```python
from build123d import *
from build123d.topology import SkipClean

# Parameters (mm, degrees)
SKETCH1_R           = 37.25
BOSS_EXTRUDE1_DEPTH = 1.2
SKETCH2_R           = 20.1
SKETCH2_W           = 26.3
SKETCH2_H           = 19.35
SKETCH2_W_2         = 15.8
SKETCH2_H_2         = 1.8
BOSS_EXTRUDE3_DEPTH = 2
SKETCH2_5_R         = 22.5
SKETCH2_5_R_2       = 20.1
BOSS_EXTRUDE4_DEPTH = 5.6
SKETCH2_7_R         = 22.5
SKETCH2_7_R_2       = 20.1
SKETCH2_7_W         = 26.3
SKETCH2_7_H         = 19.35
SKETCH2_7_W_2       = 15.8
SKETCH2_7_H_2       = 1.8
CUT_EXTRUDE1_DEPTH  = 55.800866781
CUT_EXTRUDE2_DEPTH  = 54.52919764
SKETCH8_R           = 1.5
CUT_EXTRUDE3_DEPTH  = 55.283837374
CUT_EXTRUDE4_DEPTH  = 54.52919764
CUT_EXTRUDE5_REACH  = 74.76


with BuildPart() as part:
    # Sketch1 → Boss-Extrude1 (new body)
    with BuildSketch(Plane(origin=(0, 0, 0), x_dir=(1, 0, 0), z_dir=(0, 1, 0))):
        with Locations(Location((0, 0, 0), (0, 0, 270))):
            Circle(SKETCH1_R)
    extrude(amount=BOSS_EXTRUDE1_DEPTH)

    # Sketch2 → Boss-Extrude3 (add)
    # profile 1 of 3: a face of its own
    with BuildSketch(Plane(origin=(0, 1.2, 0), x_dir=(1, 0, 0), z_dir=(0, 1, 0))):
        with Locations(Location((0, 0, 0), (0, 0, 270))):
            Circle(SKETCH2_R)
        with Locations((-2.45, 1.2)):
            Rectangle(SKETCH2_W, SKETCH2_H, mode=Mode.SUBTRACT)
    # profile 2 of 3: a face of its own
    with BuildSketch(Plane(origin=(0, 1.2, 0), x_dir=(1, 0, 0), z_dir=(0, 1, 0))):
        with Locations((0, 7.175)):
            Rectangle(SKETCH2_W_2, SKETCH2_H_2)
    # profile 3 of 3: a face of its own
    with BuildSketch(Plane(origin=(0, 1.2, 0), x_dir=(1, 0, 0), z_dir=(0, 1, 0))):
        with Locations((0, -7.175)):
            Rectangle(SKETCH2_W_2, SKETCH2_H_2)
    extrude(amount=BOSS_EXTRUDE3_DEPTH)

    # Sketch2<5> → Boss-Extrude4 (add)
    with BuildSketch(Plane(origin=(0, 1.2, 0), x_dir=(1, 0, 0), z_dir=(0, 1, 0))):
        with Locations(Location((0, 0, 0), (0, 0, 270))):
            Circle(SKETCH2_5_R)
        with Locations(Location((0, 0, 0), (0, 0, 270))):
            Circle(SKETCH2_5_R_2, mode=Mode.SUBTRACT)
    extrude(amount=BOSS_EXTRUDE4_DEPTH)


with BuildPart() as body_2:
    # Loft1: read off the stored shape, not the designer's step
    # Loft1 outline → Loft1 (revolve)
    with BuildSketch(Plane.XY):
        Polygon((0, 16.3), (0, 1.2), (37.25, 1.2), (24.5, 16.3), align=None)
    revolve(axis=Axis((0, 0, 0), (0, 1, 0)))

    # Sketch2<7> → Cut-Extrude1 (cut, through all)
    # profile 1 of 5: a face of its own
    with BuildSketch(Plane(origin=(0, 1.2, 0), x_dir=(1, 0, 0), z_dir=(0, 1, 0))):
        with Locations(Location((0, 0, 0), (0, 0, 90))):
            Circle(SKETCH2_7_R)
        with Locations(Location((0, 0, 0), (0, 0, 270))):
            Circle(SKETCH2_7_R_2, mode=Mode.SUBTRACT)
    # profile 2 of 5: a face of its own
    with BuildSketch(Plane(origin=(0, 1.2, 0), x_dir=(1, 0, 0), z_dir=(0, 1, 0))):
        with Locations(Location((0, 0, 0), (0, 0, 270))):
            Circle(SKETCH2_7_R_2)
        with Locations((-2.45, 1.2)):
            Rectangle(SKETCH2_7_W, SKETCH2_7_H, mode=Mode.SUBTRACT)
    # profile 3 of 5: a face of its own
    with BuildSketch(Plane(origin=(0, 1.2, 0), x_dir=(1, 0, 0), z_dir=(0, 1, 0))):
        with Locations((-2.45, 1.2)):
            Rectangle(SKETCH2_7_W, SKETCH2_7_H)
        with Locations((0, 7.175)):
            Rectangle(SKETCH2_7_W_2, SKETCH2_7_H_2, mode=Mode.SUBTRACT)
        with Locations((0, -7.175)):
            Rectangle(SKETCH2_7_W_2, SKETCH2_7_H_2, mode=Mode.SUBTRACT)
    # profile 4 of 5: a face of its own
    with BuildSketch(Plane(origin=(0, 1.2, 0), x_dir=(1, 0, 0), z_dir=(0, 1, 0))):
        with Locations((0, 7.175)):
            Rectangle(SKETCH2_7_W_2, SKETCH2_7_H_2)
    # profile 5 of 5: a face of its own
    with BuildSketch(Plane(origin=(0, 1.2, 0), x_dir=(1, 0, 0), z_dir=(0, 1, 0))):
        with Locations((0, -7.175)):
            Rectangle(SKETCH2_7_W_2, SKETCH2_7_H_2)
    extrude(amount=CUT_EXTRUDE1_DEPTH, mode=Mode.SUBTRACT)


with BuildPart() as part_1:
    add(part.part)

    # Combine1: union body 2
    add(body_2.part)

    # Sketch7 → Cut-Extrude2 (cut, through all)
    with BuildSketch(Plane(origin=(0, 6.8, 0), x_dir=(1, 0, 0), z_dir=(0, 1, 0))):
        with BuildLine():
            Line((-7.9, 10.875), (-7.9, -8.475))
            Line((-7.9, -8.475), (-20.842849493, -8.475))
            ThreePointArc((-20.842849493, -8.475), (-22.460675412, 1.329684188), (-19.69731898, 10.875))
            Line((-19.69731898, 10.875), (-7.9, 10.875))
        make_face()
    extrude(amount=-CUT_EXTRUDE2_DEPTH, mode=Mode.SUBTRACT)

    # Sketch8 → Cut-Extrude3 (cut, through all)
    with BuildSketch(Plane(origin=(0, 3.2, 0), x_dir=(1, 0, 0), z_dir=(0, 1, 0))):
        with Locations(Location((0, 14, 0), (0, 0, 270))):
            Circle(SKETCH8_R)
        with Locations(Location((0, -14, 0), (0, 0, 270))):
            Circle(SKETCH8_R)
    extrude(amount=-CUT_EXTRUDE3_DEPTH, mode=Mode.SUBTRACT)

    # Sketch9 → Cut-Extrude4 (cut, through all)
    with SkipClean():  # the faces are left unmerged after this step: merging them gives an invalid solid
        with BuildSketch(Plane(origin=(0, 6.8, 0), x_dir=(1, 0, 0), z_dir=(0, 1, 0))):
            with BuildLine():
                Line((7.9, 10.875), (7.9, -8.475))
                Line((7.9, -8.475), (20.842849493, -8.475))
                ThreePointArc((20.842849493, -8.475), (22.460675412, 1.329684188), (19.69731898, 10.875))
                Line((19.69731898, 10.875), (7.9, 10.875))
            make_face()
        extrude(amount=-CUT_EXTRUDE4_DEPTH, mode=Mode.SUBTRACT)

    # Chamfer1: read off the stored shape, not the designer's step
    # Chamfer1 outline → Chamfer1 (revolve, cut)
    with SkipClean():  # the faces are left unmerged after this step: merging them gives an invalid solid
        with BuildSketch(Plane.XY):
            Polygon((37.25, 1.806111173), (36.738217387, 1.806111173), (37.25, 0.4), align=None)
        revolve(axis=Axis((0, 0, 0), (0, 1, 0)), mode=Mode.SUBTRACT)

    # Cut-Extrude5: up to this cone (the profile starts outside it)
    with SkipClean():  # the faces are left unmerged after this step: merging them gives an invalid solid
        cut_extrude5_end = Plane(origin=(0, 13.007369, 0), z_dir=(0, -1, 0)).offset(-31.6883035) * Cone(1e-06, 112.896593677, 133.704984453, align=(Align.CENTER, Align.CENTER, Align.MIN), mode=Mode.PRIVATE)
        # Sketch10 → Cut-Extrude5 (cut, up to the surface)
        with BuildSketch(Plane(origin=(22.337472556, 18.861110933, 0), x_dir=(0, 0, -1), z_dir=(0.7640576290946525, 0.6451479980766108, 0)), mode=Mode.PRIVATE) as cut_extrude5_sk1:
            Polygon((0, -5.351986599), (-2, -8.816088214), (2, -8.816088214), align=None)
        cut_extrude5_tool1 = extrude(cut_extrude5_sk1.sketch, amount=-CUT_EXTRUDE5_REACH, mode=Mode.PRIVATE) - cut_extrude5_end
        add(cut_extrude5_tool1.solids().sort_by_distance((27.280201, 13.007369, 0))[0], mode=Mode.SUBTRACT)


solid = part_1.part
```
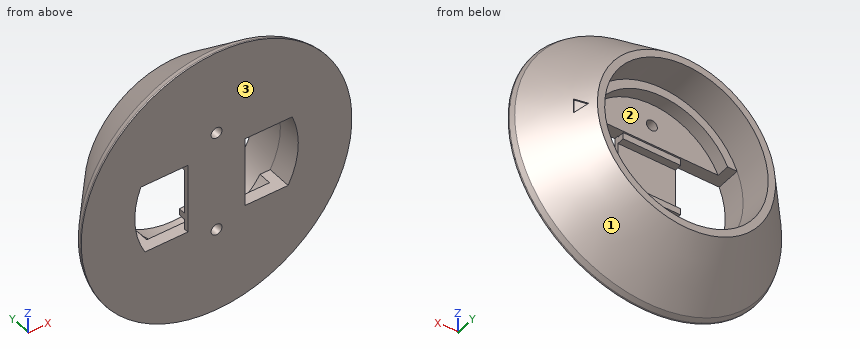
Read the model definition and answer for the solid it produces. Units are mm, in the model's axes. Face numbers are marked on the shaded views. Round coordinates to 2 decimals unless told otherwise and drop trailing zeros. Write each loop counter-clockwise with the first axis right and the second up, starting at its lowest first coordinate (ties: lowest second). Pieces come first, ordered by that corner, then holes. Notation, with made-up numbers: M -10.5,24.25 L 5.5,24.25 A21 cw 5.5,42.25 Z; hole C 69,78.5 d3. An arc over 180 degrees is marked long. One line per item, written item: value.
Q1. Find section A-A on x = 0. Count the separate pieces of the cut face and the enclosed holes in it, plus the area to 3 significant figures.
Data:
separate pieces: 3
enclosed holes: 0
area: 398 mm2
Q2. For a pull along X with two mould halves and no side action, classify the marked faces 1, 2 and 3 as +X half, -X half, draft (parallel to the pull), parting line (faces both ways), or undercut.
Data:
face 1: parting line
face 2: undercut
face 3: draft
Q3. Find section B-B on y = 8.25. Write down the section's boundary in (x, z).
Data:
outline: C 0,0 d62.59; hole C 0,0 d45
Q4. Flat-ended cylindrical pins translate along their axes: pin 1 Ø2 at (x, y) = (1, 2) entering from +Z; pin 2 Ø2 at (x, y) = (-23.5, 10.5) entering from +Z; pin 3 Ø5 at (x, z) = (0, -14) entering from +Y. Find the tip coordinate at first contact, or state that the pin passes through.
Data:
pin 1: z = 37.02
pin 2: z = 19.5
pin 3: y = 3.2
Q5. Straight lines are drawn through the part: line 1 (X direction, y = 2.25, z = 8); line 2 (Z direction, x = 14, y = 7.25); line 3 (Y direction, x = -3.5, z = 22). For each, find the intervals that lie inside material, in ascending order. Write a range as [from, to].
Data:
line 1: [-35.47, -21.03], [-7.9, 7.9], [21.03, 35.47]
line 2: [-28.93, -17.61], [17.61, 28.93]
line 3: [0, 6.8]
